Source: CAD feature listing. Evaluate the final solid. Frame: model axes, mm. A direction names the side the tool comes from. Coordinates: 2 decimals unless noted, no trailing zeros. Order: outer loops, then holes, each group sorted by start corner. A loop starts at its lowest first (then second) coordinate and runs counter-clockwise, first axis right, second up.
```python
from build123d import *

# Parameters (mm, degrees)
F1_DEPTH  = 80
F8_DEPTH  = 2.5
F9_T      = -4
F10_D     = 5
F14_D     = 5
F15_D     = 5
F15_DEPTH = 51.001


with BuildPart() as f1:
    # F0 (on Top) → F1 (new body)
    with BuildSketch(Plane.XY):
        Polygon((44, -43), (44, 43), (37, 43), (-37, 43), (-44, 43), (-44, -43), (-37, -43), (37, -43), align=None)
    extrude(amount=F1_DEPTH)

    # F7 (on 3pt) → F8 (join)
    with BuildSketch(Plane.XY.offset(21.5)):
        Polygon((-47.5, 39.5), (-51, 43), (-51, 36), align=None)
        Polygon((-51, 36), (-44, 36), (-47.5, 39.5), align=None)
        Polygon((-44, 36), (-44, 43), (-47.5, 39.5), align=None)
        Polygon((-47.5, 39.5), (-44, 43), (-51, 43), align=None)
        Polygon((51, 43), (44, 43), (47.5, 39.5), align=None)
        Polygon((47.5, 39.5), (44, 36), (51, 36), align=None)
        Polygon((51, 36), (51, 43), (47.5, 39.5), align=None)
        Polygon((47.5, 39.5), (44, 43), (44, 36), align=None)
        Polygon((47.5, -39.5), (44, -43), (51, -43), align=None)
        Polygon((51, -36), (44, -36), (47.5, -39.5), align=None)
        Polygon((51, -43), (51, -36), (47.5, -39.5), align=None)
        Polygon((47.5, -39.5), (44, -36), (44, -43), align=None)
        Polygon((-44, -43), (-44, -36), (-47.5, -39.5), align=None)
        Polygon((-47.5, -39.5), (-44, -36), (-51, -36), align=None)
        Polygon((-51, -43), (-47.5, -39.5), (-51, -36), align=None)
        Polygon((-51, -43), (-44, -43), (-47.5, -39.5), align=None)
    extrude(amount=F8_DEPTH)

    # F9
    f9_openings = [f1.faces().sort_by_distance(p)[0] for p in [
        (0, 0, 0),
    ]]
    offset(amount=F9_T, openings=f9_openings, kind=Kind.INTERSECTION)

    # F10 (through all)
    with Locations(Plane(origin=(0, 0, 21.5), x_dir=(1, 0, 0), z_dir=(0, 0, -1))):
        with Locations((47.5, 39.5), (47.5, -39.5), (-47.5, -39.5), (-47.5, 39.5)):
            Hole(F10_D / 2)

    # F14 (through all)
    with Locations(Plane(origin=(44, 0, 0), x_dir=(0, -1, 0), z_dir=(1, 0, 0))):
        with Locations((0, -38.1846800447)):
            Hole(F14_D / 2)

    # F15 (through all, one way)
    with BuildSketch(Plane.YZ):
        with Locations((0, 38.2145792246)):
            Circle(F15_D / 2)
    extrude(amount=-F15_DEPTH, mode=Mode.SUBTRACT)


solid = f1.part
```
Q1. Set-up query: faces 3 (the flat face through (-50, 41, 21.5)), 4 (the flat face through (1, 39, 37)), 5 (the flat face through (45, 41, 21.5)). Return all of +Z, -Z, +X, -X, +Y, -Y with unobstructed straight access to the full face (end or side cutting, diameter ignored); none if empty.
Solutions:
face 3: -Z, -X, +Y, -Y
face 4: -Z
face 5: -Z, +X, +Y, -Y
Q2. Section query B-B on x = -47.5. Output: boundary loops of the cut face in (y, z), plus the area to 3 significant figures.
Solutions:
outline: (-43, 21.5) - (-42, 21.5) - (-42, 24) - (-43, 24) - close; (-37, 21.5) - (-36, 21.5) - (-36, 24) - (-37, 24) - close; (36, 21.5) - (37, 21.5) - (37, 24) - (36, 24) - close; (42, 21.5) - (43, 21.5) - (43, 24) - (42, 24) - close
area: 10.0 mm2
Q3. Section query A-A on y = 0. Output: boundary loops of the cut face in (x, z).
Solutions:
outline: (-44, 0) - (-40, 0) - (-40, 35.68) - (-44, 35.68) - close; (-44, 40.71) - (-40, 40.71) - (-40, 76) - (40, 76) - (40, 40.68) - (44, 40.68) - (44, 80) - (-44, 80) - close; (40, 0) - (44, 0) - (44, 35.68) - (40, 35.68) - close
Q4. Pin query (flat end, axial travel): P1, Ø4, axis at y = 5, z = 59.5, coming from the +X side; P2, Ø7.5, axis at x = -48.5, y = -38.5, coming from the -Z side; P3, Ø23, axis at y = -10.5, z = 24, coming from the -X side; P4, Ø3, axis at x = -47.5, y = -39.5, coming from the +Z side. Return the tip coordinate at first contact, or that it passes through.
Solutions:
P1: stops at x = 44
P2: stops at z = 21.5
P3: stops at x = -44
P4: passes through
Q5. Section query C-C on z = 67.5. Output: boundary loops of the cut face in (x, y), plus the area to 3 significant figures.
Solutions:
outline: (-44, -43) - (44, -43) - (44, 43) - (-44, 43) - close; hole (-40, -39) - (40, -39) - (40, 39) - (-40, 39) - close
area: 1,330 mm2
Q6. Pull-direction query (Y, two-part tool) for faces 1 (the cylindrical face through (41.972, -0.542, 40.625)), 2 (the flat face through (-51, -39, 23)); classes: pulls with the +Y half, pulls with the -Y half, needs draft (parallel to the pull), parting line crosses it, or undercut.
Solutions:
face 1: undercut
face 2: needs draft
Q7. Section query D-D on y = -22. Output: boundary loops of the cut face in (x, z), plus the area to 3 significant figures.
Solutions:
outline: (-44, 0) - (-40, 0) - (-40, 76) - (40, 76) - (40, 0) - (44, 0) - (44, 80) - (-44, 80) - close
area: 960 mm2
Q8. Material intervals for line 1 along X through (y, z) = (-39.5, 23.4); line 2 along Y through (x, z) = (47.5, 22.05); line 3 along X through (y, z) = (-37, 45.5), sorted ascending.
Solutions:
line 1: x = -51 to -50, -45 to 45, 50 to 51
line 2: y = -43 to -42, -37 to -36, 36 to 37, 42 to 43
line 3: x = -44 to -40, 40 to 44
